Autodesk Inventor part; units mm, degrees
ref_plane "schraube_st_XY" through (0, 0, -3.5) normal (0, 0, 1) x (1, 0, 0)
ref_plane "schraube_st_YZ" through (0, 0, -3.5) normal (1, 0, 0) x (0, 1, 0)
ref_plane "schraube_st_ZX" through (0, 0, -3.5) normal (0, 1, 0) x (0, 0, 1)
sketch "Sketch_1" plane through (0, 0, 0) normal (0, 0, 1) x (1, 0, 0)
  line L0 (-4, -2.3094) -> (0, -4.6188)
  line L1 (0, -4.6188) -> (4, -2.3094)
  line L2 (4, -2.3094) -> (4, 2.3094)
  line L3 (4, 2.3094) -> (0, 4.6188)
  line L4 (0, 4.6188) -> (-4, 2.3094)
  line L5 (-4, 2.3094) -> (-4, -2.3094)
extrude "Extrusion1" add sketch "Sketch_1" against normal blind 3
sketch "Sketch_2" plane through (0, 0, 0) normal (1, 0, 0) x (0, 0, -1)
  line L0 (3.5, 0) -> (3, 0)
  line L1 (3, 0) -> (3, 3.45)
  line L2 (3, 3.45) -> (3.5, 3.45)
  line L3 (3.5, 3.45) -> (3.5, 0)
  line L4 (3.5, 0) -> (3, 0)
revolve "Revolution1" add sketch "Sketch_2" angle 360 about axis through (0, 0, -3.5) along (0, 0, -1)
sketch "Sketch_3" plane through (0, 0, 0) normal (1, 0, 0) x (0, 0, -1)
  line L0 (15.5, 0) -> (3.5, 0)
  line L1 (3.5, 0) -> (3.5, 2.5)
  line L2 (3.5, 2.5) -> (15.0095, 2.5)
  line L3 (15.0095, 2.5) -> (15.5, 2.0095)
  line L4 (15.5, 2.0095) -> (15.5, 0)
  line L5 (15.5, 0) -> (3.5, 0)
revolve "Revolution2" add sketch "Sketch_3" angle 360 about axis through (0, 0, -15.5) along (0, 0, -1)
thread "Thread1"
sketch "Sketch_4" plane through (0, 0, 0) normal (1, 0, 0) x (0, 0, -1)
  line L0 (50, 0) -> (-50, 0)
  line L1 (-2, 3.9903) -> (0, 3.9903)
  line L2 (0, 3.9903) -> (0.6285, 4.6188)
  line L3 (0.6285, 4.6188) -> (0.6285, 6.6188)
  line L4 (0.6285, 6.6188) -> (-2, 6.6188)
  line L5 (-2, 6.6188) -> (-2, 3.9903)
revolve "Revolution3" cut sketch "Sketch_4" angle 360 about axis through (0, 0, -50) along (0, 0, -1)
ref_plane "schraube_st_XY" through (0, 0, -3.5) normal (0, 0, 1) x (1, 0, 0)
ref_plane "schraube_st_YZ" through (0, 0, -3.5) normal (1, 0, 0) x (0, 1, 0)
ref_plane "schraube_st_ZX" through (0, 0, -3.5) normal (0, 1, 0) x (0, 0, 1)
properties part number "61581400_5"
CAD build for the part. Positions are in the model's coordinates, mm. A direction names the side the tool comes from. Give positions to 0.01 mm unless a question says otherwise; leave off trailing zeros. Order: outer loops, then holes, each group sorted by start corner. A loop starts at its lowest first (then second) coordinate and runs counter-clockwise, first axis right, second up.
(1) Saw through at B-B, the plane z = -6.25. Give the cut face in (x, y).
(2) Flat gauge pins, fed straight in: pin 1 (1 mm diameter, centred on x = -1.5, z = -14, fed in from -Y); pin 2 (2 mm diameter, centred on x = 1.5, z = -8.5, fed in from +Y); pin 3 (1.5 mm diameter, centred on x = 1.5, y = -2.5, fed in from -Z). Where does each tip first touch, or does it go through?
(3) Drill centre lines: L1, parallel to Z at x = -3.25, y = -1.25; L2, parallel to Z at x = -1, y = -2.75; L3, parallel to X at y = -1.5, z = -8.75. Where is each one in solid material? Low to high.
(4) Tool access for faces 1 (the cylindrical face through (-2.44, -0.54, -9.34)), 2 (the flat face through (4, 0, -1)): list every direction of +Z, -Z, +X, -X, +Y, -Y with a clear straight run to the whole face (end or side of a thin tool).
Results found:
1. outline: circle Ø5 at (0, 0)
2. pin 1: stops at y = -2.29
2. pin 2: stops at y = 2.45
2. pin 3: stops at z = -15.34
3. L1: z = -3 to 0
3. L2: z = -3.5 to 0
3. L3: x = -2 to 2
4. face 1: -Z
4. face 2: +Z, -Z, +X, +Y, -Y
